```python
from build123d import *

# Parameters (mm, degrees)
SKETCH1_W           = 97
SKETCH1_H           = 30
BOSS_EXTRUDE1_DEPTH = 5
SKETCH2_R           = 2
CUT_EXTRUDE1_DEPTH  = 52.01225343
SKETCH3_W           = 5
SKETCH3_H           = 30
BOSS_EXTRUDE2_DEPTH = 50
SKETCH4_R           = 2
CUT_EXTRUDE2_DEPTH  = 113.512221558


with BuildPart() as part:
    # Sketch1 → Boss-Extrude1 (new body)
    with BuildSketch(Plane.XY):
        Rectangle(SKETCH1_W, SKETCH1_H)
    extrude(amount=BOSS_EXTRUDE1_DEPTH)

    # Sketch2 → Cut-Extrude1 (cut, through all)
    with BuildSketch(Plane.XY.offset(5)):
        with Locations((38.5, 0)):
            Circle(SKETCH2_R)
        with BuildLine():
            Line((17.292206758, 2), (31.5, 2))
            ThreePointArc((31.5, 2), (33.5, 0), (31.5, -2))
            Line((31.5, -2), (17.292206758, -2))
            ThreePointArc((17.292206758, -2), (15.292206758, 0), (17.292206758, 2))
        make_face()
    extrude(amount=-CUT_EXTRUDE1_DEPTH, mode=Mode.SUBTRACT)

    # Sketch3 → Boss-Extrude2 (add)
    with BuildSketch(Plane.XY.offset(5)):
        with Locations((-46, 0)):
            Rectangle(SKETCH3_W, SKETCH3_H)
    extrude(amount=BOSS_EXTRUDE2_DEPTH)

    # Sketch4 → Cut-Extrude2 (cut, through all)
    with BuildSketch(Plane.ZY.offset(48.5)):
        with Locations(Location((15, 0, 0), (0, 0, 270))):
            Circle(SKETCH4_R)
        with Locations(Location((45, 0, 0), (0, 0, 270))):
            Circle(SKETCH4_R)
    extrude(amount=-CUT_EXTRUDE2_DEPTH, mode=Mode.SUBTRACT)


solid = part.part
```
Model file for the job. Use its own axes, mm. A direction names the side the tool comes from. Round coordinates to 2 decimals unless told otherwise and drop trailing zeros. Write each loop counter-clockwise with the first axis right and the second up, starting at its lowest first coordinate (ties: lowest second). Pieces come first, ordered by that corner, then holes. Notation, with made-up numbers: (53, 59) - (74, 59) arc R21 ccw to (74, 80) - close; hole circle Ø10 at (48.25, -30.5). An arc over 180 degrees is marked (long way). One line per item, written item: value.
(1) Cut at C-C, the plane x = 38.5. Give the cut face in (y, z), plus the area to 3 significant figures.
Values follow:
outline: (-15, 0) - (-2, 0) - (-2, 5) - (-15, 5) - close; (2, 0) - (15, 0) - (15, 5) - (2, 5) - close
area: 130 mm²
(2) Cut at D-D, the plane y = -6. Give the cut face in (x, z), plus the area to 3 significant figures.
Values follow:
outline: (-48.5, 0) - (48.5, 0) - (48.5, 5) - (-43.5, 5) - (-43.5, 55) - (-48.5, 55) - close
area: 735 mm²
(3) Cut at B-B, the plane z = 15. Give the cut face in (x, y).
Values follow:
outline: (-48.5, -15) - (-43.5, -15) - (-43.5, -2) - (-48.5, -2) - close; (-48.5, 2) - (-43.5, 2) - (-43.5, 15) - (-48.5, 15) - close
(4) Drop flat-ended pins along their axis: P1, Ø6, axis at y = -6.5, z = 26, coming from the +X side; P2, Ø2, axis at x = -1, y = -5.5, coming from the +Z side. Give the stop position or say it passes through.
Values follow:
P1: stops at x = -43.5
P2: stops at z = 5
(5) Two-plate mould, pull along X, no slides. Class faces 1 (the flat face through (-43.5, 0, 30)), 2 (the cylindrical face through (-46, 0, 17)), 3 (the cylindrical face through (36.502, 0.088, 2.535)): pulls with the +X half, pulls with the -X half, needs draft (parallel to the pull), parting line crosses it, or undercut.
Values follow:
face 1: pulls with the +X half
face 2: needs draft
face 3: undercut
(6) 3-axis set-ups, long thin cutter, end or side, ignore diameter. For faces 4 (the flat face through (2, 0, 5)), 5 (the flat face through (24, -2, 3)), 6 (the cylindrical face through (-46, 0, 43)): which of +Z, -Z, +X, -X, +Y, -Y reach the whole face in a straight line?
Values follow:
face 4: +Z, +X, +Y, -Y
face 5: +Z, -Z
face 6: +X, -X
(7) Wall check: probe 1 along Z at (x, y) = (-45.25, 0); probe 2 along X at (y, z) = (-4.75, 28.5); probe 3 along Z at (x, y) = (6.5, -8.5). Give the ranges that are in metal, low to high.
Values follow:
probe 1: z = 0 to 13, 17 to 43, 47 to 55
probe 2: x = -48.5 to -43.5
probe 3: z = 0 to 5
(8) Cut at A-A, the plane y = 0. Give the cut face in (x, z).
Values follow:
outline: (-48.5, 0) - (15.29, 0) - (15.29, 5) - (-43.5, 5) - (-43.5, 13) - (-48.5, 13) - close; (-48.5, 17) - (-43.5, 17) - (-43.5, 43) - (-48.5, 43) - close; (-48.5, 47) - (-43.5, 47) - (-43.5, 55) - (-48.5, 55) - close; (33.5, 0) - (36.5, 0) - (36.5, 5) - (33.5, 5) - close; (40.5, 0) - (48.5, 0) - (48.5, 5) - (40.5, 5) - close
